from build123d import *

# Parameters (mm, degrees)
F1_DEPTH = 3
F3_DEPTH = 1
F4_R     = 2.5
F5_DEPTH = 3
F6_DEPTH = 3


with BuildPart() as f1:
    # F0 (on Top) → F1 (new body)
    with BuildSketch(Plane.XY):
        with BuildLine():
            Line((12.5, -12.5), (12.5, 12.5))
            Line((12.5, 12.5), (-12.5, 12.5))
            Line((-12.5, 12.5), (-12.5, -12.5))
            Line((-12.5, -12.5), (-8.1482400118, -12.5))
            ThreePointArc((-8.1482400118, -12.5), (-5.8569521643, -11), (-3.5656643168, -12.5))
            Line((-3.5656643168, -12.5), (4.3517599882, -12.5))
            ThreePointArc((4.3517599882, -12.5), (6.6430478357, -11), (8.9343356832, -12.5))
            Line((8.9343356832, -12.5), (12.5, -12.5))
        make_face()
        with BuildLine():
            ThreePointArc((9.1430478357, -13.5), (9.090313618, -12.9892258908), (8.9343356832, -12.5))
            Line((8.9343356832, -12.5), (4.3517599882, -12.5))
            ThreePointArc((4.3517599882, -12.5), (6.1322737265, -15.9472657823), (9.1430478357, -13.5))
        make_face()
        with BuildLine():
            Line((4.3517599882, -12.5), (8.9343356832, -12.5))
            ThreePointArc((8.9343356832, -12.5), (6.6430478357, -11), (4.3517599882, -12.5))
        make_face()
        with BuildLine():
            ThreePointArc((-3.5656643168, -12.5), (-5.8569521643, -11), (-8.1482400118, -12.5))
            Line((-8.1482400118, -12.5), (-3.5656643168, -12.5))
        make_face()
        with BuildLine():
            Line((-3.5656643168, -12.5), (-8.1482400118, -12.5))
            ThreePointArc((-8.1482400118, -12.5), (-6.3677262735, -15.9472657823), (-3.3569521643, -13.5))
            ThreePointArc((-3.3569521643, -13.5), (-3.409686382, -12.9892258908), (-3.5656643168, -12.5))
        make_face()
    extrude(amount=F1_DEPTH)

    # F2 (on face) → F3 (cut)
    with BuildSketch(Plane.XY.offset(3)):
        with BuildLine():
            Line((5.25, 6.25), (-5.25, 6.25))
            ThreePointArc((-5.25, 6.25), (-5.5428932188, 5.5428932188), (-6.25, 5.25))
            Line((-6.25, 5.25), (-6.25, -5.25))
            ThreePointArc((-6.25, -5.25), (-5.5428932188, -5.5428932188), (-5.25, -6.25))
            Line((-5.25, -6.25), (5.25, -6.25))
            ThreePointArc((5.25, -6.25), (5.5428932188, -5.5428932188), (6.25, -5.25))
            Line((6.25, -5.25), (6.25, 5.25))
            ThreePointArc((6.25, 5.25), (5.5428932188, 5.5428932188), (5.25, 6.25))
        make_face()
        with BuildLine():
            ThreePointArc((-6.25, 5.25), (-5.5428932188, 5.5428932188), (-5.25, 6.25))
            Line((-5.25, 6.25), (-6.25, 6.25))
            Line((-6.25, 6.25), (-6.25, 5.25))
        make_face()
        with BuildLine():
            Line((-6.25, 6.25), (-5.25, 6.25))
            ThreePointArc((-5.25, 6.25), (-6.9571067812, 6.9571067812), (-6.25, 5.25))
            Line((-6.25, 5.25), (-6.25, 6.25))
        make_face()
        with BuildLine():
            ThreePointArc((7.25, 6.25), (6.25, 7.25), (5.25, 6.25))
            Line((5.25, 6.25), (6.25, 6.25))
            Line((6.25, 6.25), (6.25, 5.25))
            ThreePointArc((6.25, 5.25), (6.9571067812, 5.5428932188), (7.25, 6.25))
        make_face()
        with BuildLine():
            Line((6.25, 6.25), (5.25, 6.25))
            ThreePointArc((5.25, 6.25), (5.5428932188, 5.5428932188), (6.25, 5.25))
            Line((6.25, 5.25), (6.25, 6.25))
        make_face()
        with BuildLine():
            Line((6.25, -6.25), (6.25, -5.25))
            ThreePointArc((6.25, -5.25), (5.5428932188, -5.5428932188), (5.25, -6.25))
            Line((5.25, -6.25), (6.25, -6.25))
        make_face()
        with BuildLine():
            ThreePointArc((7.25, -6.25), (6.9571067812, -5.5428932188), (6.25, -5.25))
            Line((6.25, -5.25), (6.25, -6.25))
            Line((6.25, -6.25), (5.25, -6.25))
            ThreePointArc((5.25, -6.25), (6.25, -7.25), (7.25, -6.25))
        make_face()
        with BuildLine():
            ThreePointArc((-5.25, -6.25), (-5.5428932188, -5.5428932188), (-6.25, -5.25))
            Line((-6.25, -5.25), (-6.25, -6.25))
            Line((-6.25, -6.25), (-5.25, -6.25))
        make_face()
        with BuildLine():
            Line((-6.25, -6.25), (-6.25, -5.25))
            ThreePointArc((-6.25, -5.25), (-6.9571067812, -6.9571067812), (-5.25, -6.25))
            Line((-5.25, -6.25), (-6.25, -6.25))
        make_face()
    extrude(amount=-F3_DEPTH, mode=Mode.SUBTRACT)

    # F4 (on Top) → F5 (cut)
    with BuildSketch(Plane.XY):
        with Locations((11.5, 6.25)):
            Circle(F4_R)
        with Locations((11.5, -6.25)):
            Circle(F4_R)
    extrude(amount=-F5_DEPTH, mode=Mode.SUBTRACT)


with BuildPart() as f6:
    # F4 (on Top) → F6 (new body)
    with BuildSketch(Plane.XY):
        with Locations((11.5, 6.25)):
            Circle(F4_R)
    extrude(amount=F6_DEPTH)


with BuildPart() as f6b:
    # F4 (on Top) → F6, piece 2 (new body)
    with BuildSketch(Plane.XY):
        with Locations((11.5, -6.25)):
            Circle(F4_R)
    extrude(amount=F6_DEPTH)


with BuildPart() as f1_1:
    add(f1.part)

    # F7: cut F6b, F6
    add(f6b.part, mode=Mode.SUBTRACT)
    add(f6.part, mode=Mode.SUBTRACT)


solid = f1_1.part
Build history of the part. All positions in model axes, mm. A direction names the side the tool comes from. Round coordinates to 2 decimals unless told otherwise and drop trailing zeros. Order: outer loops, then holes, each group sorted by start corner. A loop starts at its lowest first (then second) coordinate and runs counter-clockwise, first axis right, second up. Notation, with made-up numbers: M -26,32.5 L 20,32.5 A20 ccw 20,64.5 Z; hole C -7,9.25 d11. An arc over 180 degrees is marked long. Use CSV: the item, a comma, the result in double quotes. Start each with the question number.
(1) Tool access for faces 1 (the face through (0, -2, 0)), 2 (the face through (-6.25, 0.1, 2.5)): list every direction of +Z, -Z, +X, -X, +Y, -Y with a clear straight run to the whole face (end or side of a thin tool).
(2) Cut at B-B on x = 1. List the corners of the cut face in (y, z).
(3) Flat gauge pins, fed straight in: P1, Ø1.1, axis at x = 1, z = 2.5, coming from the -Y side; P2, Ø3, axis at x = -6.25, y = -6.25, coming from the +Z side. Where does each tip first touch, or does it go through?
(4) Mould opens along Y. For faces 3 (the face through (-0.1, -6.25, 2.5)), 4 (the face through (12.5, -11, 1)), 5 (the face through (0, 12.5, 1)), 6 (the face through (-6.98, -6.933, 2.507)) say: +Y half, -Y half, draft (parallel to the pull), parting line (faces both ways), or undercut.
(5) Cut at A-A on x = 11.5. List the corners of the cut face in (y, z).
(6) Drill centre lines: probe 1 along Y at (x, z) = (11.5, 2); probe 2 along X at (y, z) = (-6.25, 1.85); probe 3 along Z at (x, y) = (5.25, -0.25). Where is each one in solid material? Low to high.
(7) Cut at C-C on z = 0.8. List the corners of the cut face in (x, y), then the cut area to 3 significant figures.
Findings:
1,face 1,"-Z, +X, -X, +Y, -Y"
1,face 2,"+Z"
2,outline,"M -12.5,0 L 12.5,0 L 12.5,3 L 6.25,3 L 6.25,2 L -6.25,2 L -6.25,3 L -12.5,3 Z"
3,P1,"stops at y = -12.5"
3,P2,"stops at z = 3"
4,face 3,"undercut"
4,face 4,"draft"
4,face 5,"+Y half"
4,face 6,"undercut"
5,outline,"M -12.5,0 L -8.75,0 L -8.75,3 L -12.5,3 Z; M -3.75,0 L 3.75,0 L 3.75,3 L -3.75,3 Z; M 8.75,0 L 12.5,0 L 12.5,3 L 8.75,3 Z"
6,probe 1,"y = -12.5 to -8.75, -3.75 to 3.75, 8.75 to 12.5"
6,probe 2,"x = -12.5 to 9"
6,probe 3,"z = 0 to 2"
7,outline,"M -12.5,-12.5 L -8.15,-12.5 A2.5 ccw long -3.57,-12.5 L 4.35,-12.5 A2.5 ccw long 8.93,-12.5 L 12.5,-12.5 L 12.5,-8.54 A2.5 cw long 12.5,-3.96 L 12.5,3.96 A2.5 cw long 12.5,8.54 L 12.5,12.5 L -12.5,12.5 Z"
7,area,"625 mm^2"
